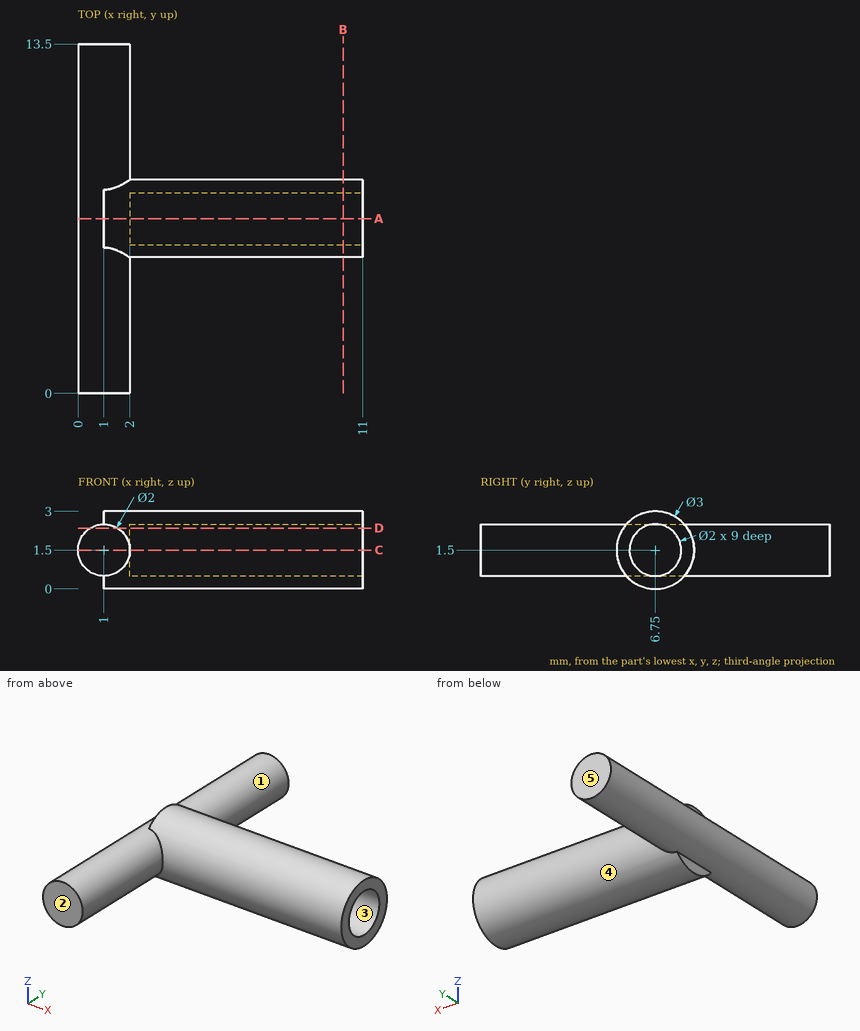
For this review, use the dimensioned drawing (mm, ordinates from the lowest corner) and the shaded views. A direction names the side the tool comes from. Round coordinates to 2 decimals unless told otherwise and drop trailing zeros. Loops run counter-clockwise (first coordinate to the right, second up) from the corner with the lowest first, then second, coordinate; pieces in that order, holes last. Notation, with made-up numbers: (75.25, 36) -> (103.25, 36) arc R29 ccw to (103.25, 68) -> close; hole circle Ø6 at (24.5, -37). An arc over 180 degrees is marked (long way). Write item = value, one per line. Start each with the question number.
Item 1: Take a section at B-B on x = 10.25. Give the boundary of the cut face in (y, z).
Item 2: To check wall thickness, follow L1, parallel to Y at x = 4, z = 1.5; L2, parallel to Y at x = 8.5, z = 0.85; L3, parallel to X at y = 5.75, z = 2.55. State the ranges of each line that lie inside material, in increasing order.
Item 3: For the marked faces 4 and 5, list the 3-axis set-ups (+Z, -Z, +X, -X, +Y, -Y) from which the entire face can be reached by the end or side of a thin tool; tool diameter is ignored.
Item 4: Take a section at D-D on z = 2.35. Give the boundary of the cut face in (x, y), plus the area to 3 significant figures.
Item 5: Take a section at A-A on y = 6.75. Give the boundary of the cut face in (x, z).
Item 6: Take a section at C-C on z = 1.5. Give the boundary of the cut face in (x, y), plus the area to 3 significant figures.
Item 7: Mouldability with a two-part tool opening along Z and no side actions: class the marked faces 1, 2 and 3 as released by +Z, released by -Z, zero draft, split by the parting line, or undercut.
Item 8: Insertion check: pin 1 (2 mm diameter, centred on x = 7, y = 4, fed in from -Z); pin 2 (1.5 mm diameter, centred on x = 6, z = 1.5, fed in from +Y). Each pin has a flat end and moves straight along its axis. Give the tip position at first contact, or say it passes through.
Result:
q1.outline = circle Ø3 at (6.75, 1.5); hole circle Ø2 at (6.75, 1.5)
q2.L1 = 5.25 to 5.75, 7.75 to 8.25
q2.L2 = 5.4 to 5.99, 7.51 to 8.1
q2.L3 = 1 to 11
q3.face_4 = +X
q3.face_5 = +Z, -Z, +X, -X, +Y
q4.outline = (0.47, 0) -> (1.53, 0) -> (1.53, 5.51) -> (11, 5.51) -> (11, 6.22) -> (2, 6.22) -> (2, 7.28) -> (11, 7.28) -> (11, 7.99) -> (1.53, 7.99) -> (1.53, 13.5) -> (0.47, 13.5) -> close
q4.area = 28.2 mm²
q5.outline = (1, 0) -> (11, 0) -> (11, 0.5) -> (2, 0.5) -> (2, 2.5) -> (11, 2.5) -> (11, 3) -> (1, 3) -> (1, 2.5) arc R1 ccw to (1, 0.5) -> close
q6.outline = (0, 0) -> (2, 0) -> (2, 5.25) -> (11, 5.25) -> (11, 5.75) -> (2, 5.75) -> (2, 7.75) -> (11, 7.75) -> (11, 8.25) -> (2, 8.25) -> (2, 13.5) -> (0, 13.5) -> close
q6.area = 36.0 mm²
q7.face_1 = split by the parting line
q7.face_2 = zero draft
q7.face_3 = undercut
q8.pin_1 = through
q8.pin_2 = 8.25
